Read the model definition and answer for the solid it produces. Units are mm, in the model's axes. A direction names the side the tool comes from. Round coordinates to 2 decimals unless told otherwise and drop trailing zeros. Write each loop counter-clockwise with the first axis right and the second up, starting at its lowest first coordinate (ties: lowest second). Pieces come first, ordered by that corner, then holes. Notation, with made-up numbers: (-40, -15) - (17, -15) arc R10 ccw to (17, -6) - close; hole circle Ø9 at (-4, -34). An arc over 180 degrees is marked (long way). Use one line per item in the form item = value. Start each with the question number.
1) Consider line 1 along Y through (x, z) = (231, 327); line 2 along X through (y, z) = (-97, 141); line 3 along Z through (x, y) = (63.5, -227). Determine where each line is inside the solid, lowest interval first. Write a range as from..to.
2) The part is cut by section A-A, the plane z = 569. Give the vertices of the cut face in (x, y), plus the area to 3 significant figures.
3) Each of these flat-tipped pins is pushed along its axis until it touches: pin 1 (1 mm diameter, centred on y = -203, z = 434.5, fed in from -X); pin 2 (5 mm diameter, centred on x = 208.5, y = -253, fed in from +Z). Where does it stop, or does it pass through?
4) The part is cut by section C-C, the plane x = 260. Give the vertices of the cut face in (y, z), plus the area to 3 significant figures.
5) For faces 1 (the face through (163, -148, 0)), 2 (the face through (312, -148, 364)), determine the directions among +Z, -Z, +X, -X, +Y, -Y from which every point of the face is accessible in a straight line to the end or side of a thin tool.
6) The part is cut by section B-B, the plane y = -204.5. Give the vertices of the cut face in (x, z).
from build123d import *

# Parameters (mm, degrees)
F0_W     = 42.1406924725
F0_H     = 37.6295819879
F1_DEPTH = 330
F2_DEPTH = 300
F3_DEPTH = 720
F4_T     = -18


with BuildPart() as f1:
    # F0 (on Right) → F1 (new body)
    with BuildSketch(Plane.YZ):
        with Locations((-21.0703462362, 18.8147909939)):
            Rectangle(F0_W, F0_H)
    extrude(amount=F1_DEPTH)

    # F2 (add): a face of the model
    f2_faces = [f1.faces().sort_by_distance(p)[0] for p in [
        (165, 0, 18.8147909939),
    ]]
    extrude(f2_faces, amount=-F2_DEPTH)

    # F3 (add): a face of the model
    f3_faces = [f1.faces().sort_by_distance(p)[0] for p in [
        (165, -150, 0),
    ]]
    extrude(f3_faces, amount=-F3_DEPTH)

    # F4
    f4_openings = [f1.faces().sort_by_distance(p)[0] for p in [
        (0, -150, 360),
        (165, -150, 720),
    ]]
    offset(amount=F4_T, openings=f4_openings)


solid = f1.part
Geometry results:
q1.line_1 = -300..-282, -18..0
q1.line_2 = 312..330
q1.line_3 = 0..18
q2.outline = (0, -300) - (330, -300) - (330, 0) - (0, 0) - (0, -18) - (312, -18) - (312, -282) - (0, -282) - close
q2.area = 16,600 mm2
q3.pin_1 = 312
q3.pin_2 = 18
q4.outline = (-300, 0) - (0, 0) - (0, 720) - (-18, 720) - (-18, 18) - (-282, 18) - (-282, 720) - (-300, 720) - close
q4.area = 30,700 mm2
q5.face_1 = -Z, +X, -X, +Y, -Y
q5.face_2 = +Z, -X
q6.outline = (0, 0) - (330, 0) - (330, 720) - (312, 720) - (312, 18) - (0, 18) - close
